Could you check a few things on this model? Use its own coordinates, in mm. A direction names the side the tool comes from. Give positions to 0.01 mm unless a question says otherwise; leave off trailing zeros. Loops run counter-clockwise (first coordinate to the right, second up) from the corner with the lowest first, then second, coordinate; pieces in that order, holes last. Notation, with made-up numbers: (76.5, 60) - (109.5, 60) arc R21 ccw to (109.5, 88) - close; hole circle Ø4 at (-18.5, -34). An arc over 180 degrees is marked (long way). One line per item, written item: value. Start each with the question number.
Q1. I'm going to push flat-ended pins straight in: P1, Ø4, axis at x = -8.5, y = -9, coming from the -Z side; P2, Ø2, axis at y = 2.5, z = 7.5, coming from the -X side; P3, Ø3.5, axis at x = 3.5, z = 8, coming from the +Y side; P4, Ø5, axis at x = 2.75, z = 9.5, coming from the -Y side. Where does each tip first touch, or does it pass through?
Q2. I want a section at A-A (y = 7.2). Please give me the cut outline in (x, z).
Q3. I want a section at D-D (x = -6.5). Please give me the cut outline in (y, z), then the cut area to 3 significant figures.
Q4. I want a section at B-B (x = -2). Please give me the cut outline in (y, z), then the cut area to 3 significant figures.
Q5. If I drill on line 1 (Y direction, x = 2.7, z = 1.3); line 2 (X direction, y = 7.2, z = 1.55); line 3 (X direction, y = -15, z = 2.1), over which ranges is the centre line in solid material (lowest first)? Write a range as from..to.
Q6. If we mould it in two halves opening along Z, with no side actions, what happens to faces 6 (the face through (-6, -14, 3.5)), 7 (the face through (5.5, -4, 3)), 8 (the face through (2.8, 1.5, 7.9)), 9 (the face through (-2, -7, 0))? For each: released by +Z, released by -Z, zero draft, split by the parting line, or undercut.
Q7. For faces 1 (the face through (2.375, 5.736, 1.726)), 2 (the face through (0.57, 9.4, 2.02)), 3 (the face through (-5.46, -12.9, 4.01)), 4 (the face through (2.7, 3, 7.6)), 5 (the face through (4, 6, 3.5)), which set-ups out of +Z, -Z, +X, -X, +Y, -Y let a thin tool reach every point of the face, with its end or its side?
Q8. I want a section at C-C (z = 6.5). Please give me the cut outline in (x, y).
```python
from build123d import *
from OCP.BRepFilletAPI import BRepFilletAPI_MakeFillet

# Parameters (mm, degrees)
SKETCH1_R           = 1.5
BOSS_EXTRUDE1_DEPTH = 4.5
SKETCH3_R           = 1.6
BOSS_EXTRUDE2_DEPTH = 3
FILLET1_R1          = 2
FILLET1_R2          = 3
FILLET2_R           = 0.5
CUT_EXTRUDE1_DEPTH  = 1


with BuildPart() as part:
    # Sketch1 → Boss-Extrude1 (new body)
    with BuildSketch(Plane.XY):
        Polygon((-10.4, 0), (0, 0), (0, 10), (5.5, 10), (5.5, -17.8), (-10.4, -17.8), align=None)
        with Locations((2.7, 7.2)):
            Circle(SKETCH1_R, mode=Mode.SUBTRACT)
        with Locations((-7.6, -15)):
            Circle(SKETCH1_R, mode=Mode.SUBTRACT)
    extrude(amount=BOSS_EXTRUDE1_DEPTH)

    # Sketch3 → Boss-Extrude2 (add)
    with BuildSketch(Plane(origin=(0, 0, 0), x_dir=(1, 0, 0), z_dir=(0, 1, 0))):
        with BuildLine():
            Line((5.5, -4.5), (0, -4.5))
            Line((0, -4.5), (0, -9.5))
            ThreePointArc((0, -9.5), (2.75, -12.25), (5.5, -9.5))
            Line((5.5, -9.5), (5.5, -4.5))
        make_face()
        with Locations(Location((2.75, -9.5, 0), (0, 0, 270))):
            Circle(SKETCH3_R, mode=Mode.SUBTRACT)
    extrude(amount=BOSS_EXTRUDE2_DEPTH)

    # Fillet1: one fillet with a radius per group of edges: ONE call of the kernel's fillet builder (fillet() takes one radius for all edges)
    fillet1_edges_1 = [part.edges().sort_by_distance(p)[0] for p in [
        (-10.4, -17.8, 2.25),
        (5.5, 10, 2.25),
        (0, 10, 2.25),
    ]]
    fillet1_edges_2 = [part.edges().sort_by_distance(p)[0] for p in [
        (5.5, -17.8, 2.25),
    ]]
    fillet1 = BRepFilletAPI_MakeFillet(part.part.solid().wrapped)
    for e in fillet1_edges_1:
        fillet1.Add(FILLET1_R1, e.wrapped)
    for e in fillet1_edges_2:
        fillet1.Add(FILLET1_R2, e.wrapped)
    add(Compound.cast(fillet1.Shape()), mode=Mode.REPLACE)

    # Fillet2
    fillet2_edges = [part.edges().sort_by_distance(p)[0] for p in [
        (-10.4, 0, 2.25),
        (-5.2, 0, 4.5),
        (5.5, 5.5, 4.5),
        (5.5, 3, 7),
        (2.75, 3, 4.5),
        (0, 3, 7),
        (2.75, 3, 12.25),
        (-10.4, -7.9, 4.5),
        (5.5, -3.4, 0),
        (5.5, -7.4, 4.5),
        (0, 4, 0),
        (2.75, 10, 0),
        (-2.95, -17.8, 0),
        (-9.814213562, -17.214213562, 0),
        (4.914213562, 9.414213562, 0),
        (0.585786438, 9.414213562, 0),
        (4.621320344, -16.921320344, 0),
        (-2.95, -17.8, 4.5),
        (-9.814213562, -17.214213562, 4.5),
        (4.621320344, -16.921320344, 4.5),
        (0, 5.5, 4.5),
        (2.75, 10, 4.5),
        (4.914213562, 9.414213562, 4.5),
        (0.585786438, 9.414213562, 4.5),
        (-5.2, 0, 0),
        (-10.4, -7.9, 0),
    ]]
    fillet(fillet2_edges, radius=FILLET2_R)

    # Sketch6 → Cut-Extrude1 (cut)
    with BuildSketch(Plane.XY.offset(4.5)):
        with BuildLine():
            Line((-0.3, 7.2), (-0.3, 10))
            Line((-0.3, 10), (5.5, 10))
            Line((5.5, 10), (5.5, 4.2))
            Line((5.5, 4.2), (2.7, 4.2))
            ThreePointArc((2.7, 4.2), (0.578679656, 5.078679656), (-0.3, 7.2))
        make_face()
        with BuildLine():
            Line((-7.6, -12), (-10.4, -12))
            Line((-10.4, -12), (-10.4, -17.8))
            Line((-10.4, -17.8), (-4.6, -17.8))
            Line((-4.6, -17.8), (-4.6, -15))
            ThreePointArc((-4.6, -15), (-5.478679656, -12.878679656), (-7.6, -12))
        make_face()
    extrude(amount=-CUT_EXTRUDE1_DEPTH, mode=Mode.SUBTRACT)


solid = part.part
```
Worked answers:
1. P1: stops at z = 0
1. P2: stops at x = 0
1. P3: stops at y = 3
1. P4: stops at y = 0
2. outline: (0, 0.5) arc R0.5 ccw to (0.5, 0) - (1.2, 0) - (1.2, 3.5) - (0, 3.5) - close; (4.2, 0) - (5, 0) arc R0.5 ccw to (5.5, 0.5) - (5.5, 3.5) - (4.2, 3.5) - close
3. outline: (-17.8, 0.5) arc R0.5 ccw to (-17.3, 0) - (-16.02, 0) - (-16.02, 3.5) - (-17.8, 3.5) - close; (-13.98, 0) - (-0.5, 0) arc R0.5 ccw to (0, 0.5) - (0, 4) arc R0.5 ccw to (-0.5, 4.5) - (-12.21, 4.5) - (-12.21, 3.5) - (-13.98, 3.5) - close
3. area: 67.2 mm²
4. outline: (-17.8, 0.5) arc R0.5 ccw to (-17.3, 0) - (-0.5, 0) arc R0.5 ccw to (0, 0.5) - (0, 4) arc R0.5 ccw to (-0.5, 4.5) - (-17.3, 4.5) arc R0.5 ccw to (-17.8, 4) - close
4. area: 79.9 mm²
5. line 1: y = -17.79..5.7, 8.7..10
5. line 2: x = 0..1.2, 4.2..5.5
5. line 3: x = -10.4..-9.1, -6.1..5.49
6. face 6: released by +Z
6. face 7: zero draft
6. face 8: undercut
6. face 9: released by -Z
7. face 1: +Z, -Z
7. face 2: +Z, -Z, -X, +Y
7. face 3: +Z, -X, -Y
7. face 4: +Z, +X, -X, +Y
7. face 5: +Z, +X, +Y
8. outline: (0, 0) - (5.5, 0) - (5.5, 2.5) arc R0.5 ccw to (5, 3) - (0.5, 3) arc R0.5 ccw to (0, 2.5) - close
